The drawing under review shows one solid part. Ordinate dimensions are in mm from its lowest x, y, z. Give positions to 0.01 mm unless a question says otherwise; leave off trailing zeros. Write each loop counter-clockwise with the first axis right and the second up, starting at its lowest first coordinate (ties: lowest second). Pieces come first, ordered by that corner, then holes. Notation, with made-up numbers: M -5.75,57.5 L 24.25,57.5 A15 cw 24.25,66.5 Z; hole C 24,-22.75 d11. An arc over 180 degrees is marked long. Use one line per item in the form item = value. Start each with the question number.
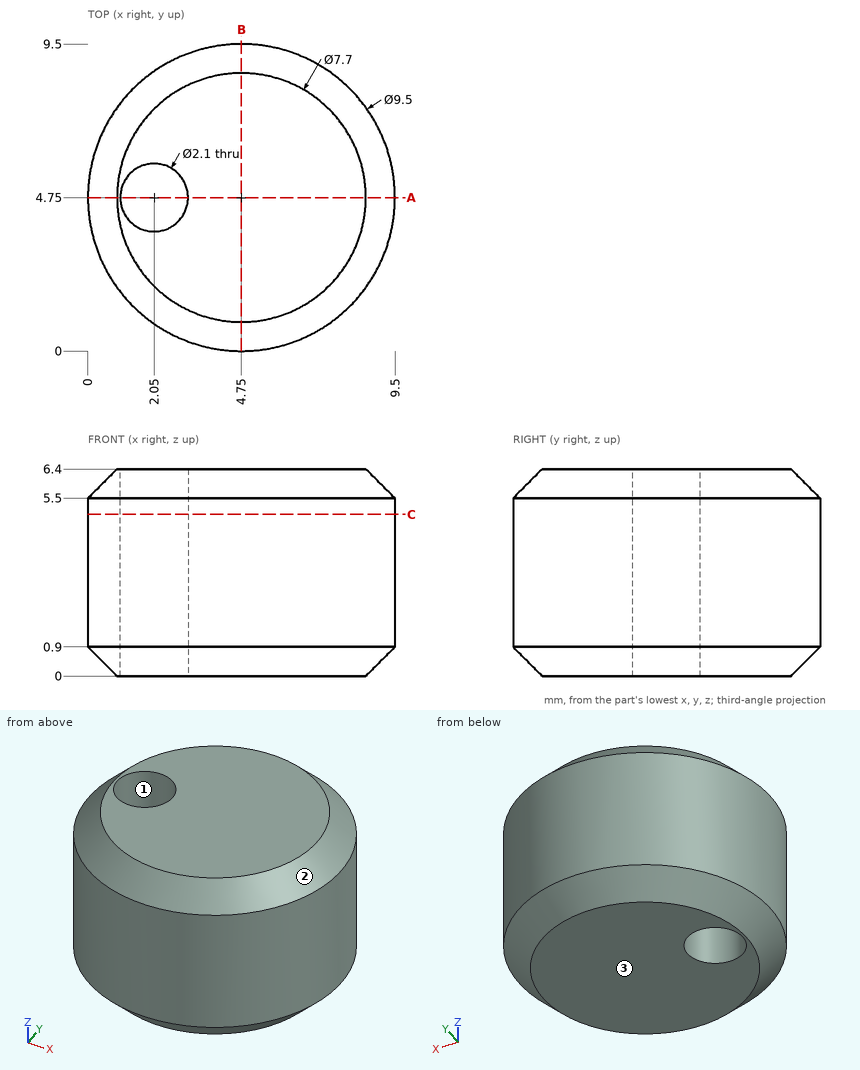
1. We need section A-A (y = 4.75). State the section outline as (x, z) points.
2. Clearance check with a flat-ended pin moving along its axis: pin 1 Ø2 at (x, z) = (2, 1.5) entering from +Y. State where the tip first meets the part, or that it passes through.
3. We need section C-C (z = 5). State the section outline as (x, y) points.
4. Draft analysis for pull direction Y (two halves, no side actions). For the marked faces 1, 2 and 3, state which applies: pulls with the +Y half, pulls with the -Y half, needs draft (parallel to the pull), parting line crosses it, or undercut.
5. We need section B-B (x = 4.75). State the section outline as (y, z) points, and give its area (3 significant figures).
6. To check wall thickness, follow L1, parallel to Y at x = 1.5, z = 2; L2, parallel to X at y = 4.5, z = 5.75; L3, parallel to Y at x = 2.05, z = 1.5. State the ranges of each line that lie inside material, in increasing order.
Answer block:
q1.outline = M 0,0.9 L 0.9,0 L 1,0 L 1,6.4 L 0.9,6.4 L 0,5.5 Z; M 3.1,0 L 8.6,0 L 9.5,0.9 L 9.5,5.5 L 8.6,6.4 L 3.1,6.4 Z
q2.pin_1 = 9.17
q3.outline = C 4.75,4.75 d9.5; hole C 2.05,4.75 d2.1
q4.face_1 = undercut
q4.face_2 = parting line crosses it
q4.face_3 = needs draft
q5.outline = M 0,0.9 L 0.9,0 L 8.6,0 L 9.5,0.9 L 9.5,5.5 L 8.6,6.4 L 0.9,6.4 L 0,5.5 Z
q5.area = 59.2 mm^2
q6.L1 = 1.29 to 3.86, 5.64 to 8.21
q6.L2 = 0.26 to 1.03, 3.07 to 9.24
q6.L3 = 0.84 to 3.7, 5.8 to 8.66
